```python
from build123d import *

# Parameters (mm, degrees)
F1_DEPTH        = 3
F2_R            = 1.7859375
F3_DEPTH        = 25
F4_T1_DEPTH     = 27.9314560345
F6_R            = 1.45
F7_DEPTH        = 25
F7_COPIES_COUNT = 4
F8_R            = 1.45
F9_DEPTH        = 25


# Not quite as in the source:
# - a fillet or chamfer that OpenCascade refuses, or shapes differently, is made with other operations: its cross-section is extruded or revolved along the edge and cut away or added
# - a pattern or mirror of a feature is missing from the dataset's text; its kind, count and spacing are read off the source's solid


with BuildPart() as f1:
    # F0 (on Front) → F1 (new body)
    with BuildSketch(Plane.XZ):
        with BuildLine():
            ThreePointArc((-17.7535207776, 10.25), (-18.9395304165, 7.8450103635), (-19.8014794389, 5.3057904246))
            add(Edge.make_bspline(
                [(-19.8014794389, 5.3057904246), (-20.454122155, 2.8700946489), (-19.9763700286, -0.7893865531), (-18.8355536126, -5.0469713795)],
                knots=[0, 0, 0, 0, 10.3977252163, 10.3977252163, 10.3977252163, 10.3977252163], degree=3))
            ThreePointArc((-18.8355536126, -5.0469713795), (-19.3331747968, 2.5452607483), (-16.8874953738, 9.75))
            Line((-16.8874953738, 9.75), (-17.7535207776, 10.25))
        make_face()
        with BuildLine():
            add(Edge.make_bspline(
                [(19.8014794389, 5.3057904246), (20.454122155, 2.8700946489), (19.9763700286, -0.7893865531), (18.8355536126, -5.0469713795)],
                knots=[0, 0, 0, 0, 10.3977252163, 10.3977252163, 10.3977252163, 10.3977252163], degree=3))
            ThreePointArc((19.8014794389, 5.3057904246), (2.6757869405, 20.3246196582), (-17.7535207776, 10.25))
            Line((-17.7535207776, 10.25), (-16.8874953738, 9.75))
            ThreePointArc((-16.8874953738, 9.75), (5.0469713795, 18.8355536126), (19.5, 0))
            ThreePointArc((19.5, 0), (19.3331747968, -2.5452607483), (18.8355536126, -5.0469713795))
        make_face()
        with BuildLine():
            ThreePointArc((-18.8355536126, -5.0469713795), (-18.015650884, -7.4623269311), (-16.8874953738, -9.75))
            ThreePointArc((-16.8874953738, -9.75), (0, -19.5), (16.8874953738, -9.75))
            ThreePointArc((16.8874953738, -9.75), (18.015650884, -7.4623269311), (18.8355536126, -5.0469713795))
            ThreePointArc((18.8355536126, -5.0469713795), (19.3331747968, -2.5452607483), (19.5, 0))
            ThreePointArc((19.5, 0), (5.0469713795, 18.8355536126), (-16.8874953738, 9.75))
            ThreePointArc((-16.8874953738, 9.75), (-19.3331747968, 2.5452607483), (-18.8355536126, -5.0469713795))
        make_face()
        with BuildLine():
            add(Edge.make_bspline(
                [(-16.8874953738, -9.75), (-15.8042909868, -11.6261650333), (-14.7498334446, -13.4051543525), (-13.7625055876, -15.1935328331)],
                knots=[0, 0, 0, 0, 6.8616960598, 6.8616960598, 6.8616960598, 6.8616960598], degree=3))
            ThreePointArc((-13.7625055876, -15.1935328331), (-0.0251276064, -20.4999846001), (13.7252177136, -15.2272255751))
            Line((13.7252177136, -15.2272255751), (14.297471583, -14.2360527984))
            add(Edge.make_bspline(
                [(16.8874953738, -9.75), (15.997662101, -11.2912364387), (15.1272281545, -12.7668954762), (14.297471583, -14.2360527984)],
                knots=[0, 0, 0, 0, 5.6367621242, 5.6367621242, 5.6367621242, 5.6367621242], degree=3))
            ThreePointArc((16.8874953738, -9.75), (0, -19.5), (-16.8874953738, -9.75))
        make_face()
        with BuildLine():
            Line((-7.5, -40), (7.5, -40))
            add(Edge.make_bspline(
                [(13.7625055876, -15.1935328331), (10.192393183, -21.6601914536), (7.5, -28.2496131611), (7.5, -40)],
                knots=[6.8616960598, 6.8616960598, 6.8616960598, 6.8616960598, 31.6731363997, 31.6731363997, 31.6731363997, 31.6731363997], degree=3))
            ThreePointArc((13.7625055876, -15.1935328331), (13.7438719752, -15.2103906304), (13.7252177136, -15.2272255751))
            ThreePointArc((13.7252177136, -15.2272255751), (-0.0251276064, -20.4999846001), (-13.7625055876, -15.1935328331))
            add(Edge.make_bspline(
                [(-13.7625055876, -15.1935328331), (-10.192393183, -21.6601914536), (-7.5, -28.2496131611), (-7.5, -40)],
                knots=[6.8616960598, 6.8616960598, 6.8616960598, 6.8616960598, 31.6731363997, 31.6731363997, 31.6731363997, 31.6731363997], degree=3))
        make_face()
        with BuildLine():
            ThreePointArc((13.7252177136, -15.2272255751), (13.7438719752, -15.2103906304), (13.7625055876, -15.1935328331))
            add(Edge.make_bspline(
                [(14.297471583, -14.2360527984), (14.1171558343, -14.5553177631), (13.9387610479, -14.8742756886), (13.7625055876, -15.1935328331)],
                knots=[5.6367621242, 5.6367621242, 5.6367621242, 5.6367621242, 6.8616960598, 6.8616960598, 6.8616960598, 6.8616960598], degree=3))
            Line((14.297471583, -14.2360527984), (13.7252177136, -15.2272255751))
        make_face()
        Polygon((7.5, -296), (7.5, -40), (-7.5, -40), (-7.5, -296), (-2.87, -296), (-2.87, -293), (2.87, -293), (2.87, -296), align=None)
    extrude(amount=F1_DEPTH)

    # F2 (on face) → F3 (cut)
    with BuildSketch(Plane.XZ.offset(3)):
        Circle(F2_R)
    extrude(amount=-F3_DEPTH, mode=Mode.SUBTRACT)

    # F4: fillet of radius 5 on 2 edges, made by hand

    # F4_s2 → F4_t1 (cut)
    with BuildSketch(Plane.XZ.offset(-12.4657280172)):
        with BuildLine():
            ThreePointArc((-7.5, -291.0137087931), (-6.1640141921, -294.4159139603), (-2.87, -296))
            Line((-2.87, -296), (-7.5, -296))
            Line((-7.5, -296), (-7.5, -291.0137087931))
        make_face()
        with BuildLine():
            ThreePointArc((7.5, -291.0137087931), (6.1640141921, -294.4159139603), (2.87, -296))
            Line((2.87, -296), (7.5, -296))
            Line((7.5, -296), (7.5, -291.0137087931))
        make_face()
    extrude(amount=F4_T1_DEPTH, mode=Mode.SUBTRACT)

    # F6 (on face) → F7 (cut)
    with BuildSketch(Plane.XZ.offset(3)):
        with Locations((0, 12)):
            Circle(F6_R)
    f7 = extrude(amount=-F7_DEPTH, mode=Mode.SUBTRACT)

    # F7_copies: F7 ×4 about axis
    f7_copies_axis = Axis((0, 0, 0), (0, 1, 0))
    for i in range(1, F7_COPIES_COUNT):
        add(f7.rotate(f7_copies_axis, i * 360 / F7_COPIES_COUNT), mode=Mode.SUBTRACT)

    # F8 (on face) → F9 (cut)
    with BuildSketch(Plane.XZ.offset(3)):
        with Locations((0, -200)):
            Circle(F8_R)
        with Locations((0, -210)):
            Circle(F8_R)
        with Locations((0, -220)):
            Circle(F8_R)
        with Locations((0, -230)):
            Circle(F8_R)
        with Locations((0, -240)):
            Circle(F8_R)
        with Locations((0, -250)):
            Circle(F8_R)
        with Locations((0, -260)):
            Circle(F8_R)
        with Locations((0, -270)):
            Circle(F8_R)
        with Locations((0, -280)):
            Circle(F8_R)
    extrude(amount=-F9_DEPTH, mode=Mode.SUBTRACT)


solid = f1.part
```
Check sheet for the modelled part. Datum: model origin and axes. Units: mm. Round coordinates to 2 decimals unless told otherwise and drop trailing zeros. Order: outer loops, then holes, each group sorted by start corner. A loop starts at its lowest first (then second) coordinate and runs counter-clockwise, first axis right, second up.
1) Scan lines: line 1 (X direction, y = -0.3, z = -260); line 2 (X direction, y = -1.3, z = -166.5); line 3 (Z direction, x = 12.5, y = -2.4). Record each from-to range of solid material in increasing order.
2) Section check B-B (y = -0.95). Give the number of separate pieces and of enclosed holes in the cut face, and give its area (3 significant figures).
3) Go/stop test with flat-tipped pins: pin 1 Ø2.5 at (x, z) = (-12, 0) entering from +Y (3 decimals); pin 2 Ø1.5 at (x, y) = (7.5, -0.5) entering from -Z. Record where each tip stops, or that it passes through.
4) Section check A-A (z = -103.5). Record the boundary of the cut face in (x, y).
Result:
1. line 1: x = -7.5 to -1.45, 1.45 to 7.5
1. line 2: x = -7.5 to 7.5
1. line 3: z = -17.57 to -1.36, 1.36 to 16.25
2. separate pieces: 1
2. enclosed holes: 14
2. area: 5,370 mm2
3. pin 1: passes through
3. pin 2: stops at z = -293.65
4. outline: (-7.5, -3) - (7.5, -3) - (7.5, 0) - (-7.5, 0) - close
